Part model, mm, in its own coordinate system. Give positions to 0.01 mm unless a question says otherwise; leave off trailing zeros. Order: outer loops, then holes, each group sorted by start corner. A loop starts at its lowest first (then second) coordinate and runs counter-clockwise, first axis right, second up. Notation, with made-up numbers: (66.25, -4.75) -> (105.25, -4.75) arc R25 cw to (105.25, 16.25) -> close; hole circle Ø8 at (-13, -10). An arc over 180 degrees is marked (long way). Write item = value, one per line. Start each with the question number.
(1) Two-plate mould, pull along X, no slides. Class faces 1 (the cylindrical face through (8.767, 11.224, -16.856)), 2 (the flat face through (14, 8.636, 14)), 3 (the cylindrical face through (9.139, 7.04, -14.334)): pulls with the +X half, pulls with the -X half, needs draft (parallel to the pull), parting line crosses it, or undercut.
(2) Saw through at B-B, the plane z = 0. List the corners of the cut face in (x, y), then the cut area to 3 significant figures.
(3) Saw through at D-D, the plane x = -18. List the corners of the cut face in (y, z).
(4) Saw through at C-C, the plane y = 7. List the corners of the cut face in (x, z), then the cut area to 3 significant figures.
(5) Flat gauge pins, fed straight in: pin 1 (4 mm diameter, centred on x = -14, y = 11, fed in from +Z); pin 2 (5 mm diameter, centred on x = -1.5, y = 2, fed in from +Z); pin 3 (5 mm diameter, centred on y = 7.5, z = -11, fed in from -X). Where does each tip first touch, or does it go through?
(6) Saw through at A-A, the plane x = 0. List the corners of the cut face in (y, z).
(7) Probe line 1 along X through (y, z) = (10, 0); line 2 along Z through (x, y) = (0, 8.5). List the from-to ranges inside material, lowest first. Write a range as from..to.
Autodesk Inventor part; units mm, degrees
ref_plane "YZ Plane" through (0, 0, 0) normal (1, 0, 0) x (0, 1, 0)
ref_plane "XZ Plane" through (0, 0, 0) normal (0, 1, 0) x (-1, 0, 0)
ref_plane "XY Plane" through (0, 0, 0) normal (0, 0, 1) x (1, 0, 0)
sketch "Sketch1" plane through (0, 0, 0) normal (0, 1, 0) x (-1, 0, 0)
  circle A0 centre (0, 0) radius 25.8445
  dimension "d0" = 51.689
extrude "Extrusion1" add sketch "Sketch1" along normal blind 8.636
sketch "Sketch2" plane through (0, 8.636, 0) normal (0, 1, 0) x (1, 0, 0)
  circle A0 centre (0, 0) radius 19
  dimension "d3" = 37.9999
extrude "Extrusion2" add sketch "Sketch2" along normal blind 5.25
sketch "Sketch3" plane through (0, 13.886, 0) normal (0, 1, 0) x (1, 0, 0)
  circle A0 centre (0, 0) radius 17
  dimension "d6" = 33.9999
extrude "Extrusion3" cut sketch "Sketch3" against normal through all
thread "Thread2"
properties part number "38mm to SM2" material "Aluminum 6061-AHC"
Results list:
q1.face_1 = parting line crosses it
q1.face_2 = needs draft
q1.face_3 = undercut
q2.outline = (-25.84, 0) -> (-17, 0) -> (-17, 13.89) -> (-19, 13.89) -> (-19, 8.64) -> (-25.84, 8.64) -> close; (17, 0) -> (25.84, 0) -> (25.84, 8.64) -> (19, 8.64) -> (19, 13.89) -> (17, 13.89) -> close
q2.area = 174 mm^2
q3.outline = (0, -18.55) -> (8.64, -18.55) -> (8.64, -6.08) -> (13.89, -6.08) -> (13.89, 6.08) -> (8.64, 6.08) -> (8.64, 18.55) -> (0, 18.55) -> close
q4.outline = circle Ø51.69 at (0, 0); hole circle Ø34 at (0, 0)
q4.area = 1,190 mm^2
q5.pin_1 = 14.73
q5.pin_2 = 25.84
q5.pin_3 = -24.41
q6.outline = (0, -25.84) -> (8.64, -25.84) -> (8.64, -19) -> (13.89, -19) -> (13.89, -17) -> (0, -17) -> close; (0, 17) -> (13.89, 17) -> (13.89, 19) -> (8.64, 19) -> (8.64, 25.84) -> (0, 25.84) -> close
q7.line_1 = -19..-17, 17..19
q7.line_2 = -25.84..-17, 17..25.84
